Autodesk Inventor part; units mm, degrees
ref_plane "YZ Plane" through (0, 0, 0) normal (1, 0, 0) x (0, 1, 0)
ref_plane "XZ Plane" through (0, 0, 0) normal (0, 1, 0) x (-1, 0, 0)
ref_plane "XY Plane" through (0, 0, 0) normal (0, 0, 1) x (1, 0, 0)
sketch "Sketch1" plane through (0, 0, 0) normal (0, 1, 0) x (-1, 0, 0)
  line L0 (41.8301, 96.0131) -> (-38.1699, 96.0131)
  line L1 (-38.1699, 96.0131) -> (-38.1699, -53.9869)
  line L2 (-38.1699, -53.9869) -> (41.8301, -53.9869)
  line L3 (41.8301, -53.9869) -> (41.8301, 96.0131)
  line L4 (41.8301, 81.0131) -> (-35.1699, 81.0131)
  line L5 (-35.1699, 81.0131) -> (-35.1699, -38.9869)
  line L6 (-35.1699, -38.9869) -> (41.8301, -38.9869)
  line L7 (41.8301, -38.9869) -> (41.8301, 81.0131)
  point P0 (0, 0)
  dimension "d0" = 80
  dimension "d1" = 150
  dimension "d2" = 15
  dimension "d3" = 15
  dimension "d4" = 3
extrude "Extrusion1" add sketch "Sketch1" along normal blind 15 contours L3 L4 L5 L6 L2 L1 L0
sketch "Sketch2" plane through (0, 15, 0) normal (0, 1, 0) x (1, 0, 0)
  line L0 (-41.8301, -96.0131) -> (38.1699, -96.0131)
  line L1 (-38.8301, -96.0131) -> (35.1699, -96.0131)
  line L2 (35.1699, -96.0131) -> (35.1699, -85.0131)
  line L3 (35.1699, -85.0131) -> (-38.8301, -85.0131)
  line L4 (-38.8301, -85.0131) -> (-38.8301, -96.0131)
  line L5 (38.1699, 53.9869) -> (-41.8301, 53.9869)
  line L6 (-38.8301, 53.9869) -> (35.1699, 53.9869)
  line L7 (35.1699, 53.9869) -> (35.1699, 42.9869)
  line L8 (35.1699, 42.9869) -> (-38.8301, 42.9869)
  line L9 (-38.8301, 42.9869) -> (-38.8301, 53.9869)
  line L10 (35.1699, -81.0131) -> (-41.8301, -81.0131)
  line L11 (-41.8301, 38.9869) -> (35.1699, 38.9869)
  line L12 (-41.8301, 53.9869) -> (-41.8301, 38.9869)
  point P0 (0, 0)
  point P1 (35.1699, -96.0131)
  dimension "d7" = 4
  dimension "d8" = 4
  dimension "d9" = 3
extrude "Extrusion2" cut sketch "Sketch2" against normal blind 11
sketch "Sketch3" plane through (-41.8301, 0, -53.9869) normal (-1, 0, 0) x (0, 0, 1)
  circle A0 centre (5, 10) radius 1.4
  circle A1 centre (145, 10) radius 1.4
  line L0 (11, 15) -> (11, 4)
  line L1 (11, 4) -> (0, 4)
  line L2 (139, 15) -> (139, 4)
  line L3 (150, 4) -> (139, 4)
  point P0 (53.9869, 0)
  dimension "d12" = 2.8
  dimension "d13" = 2.8
  dimension "d14" = 6
  dimension "d15" = 6
  dimension "d16" = 6
  dimension "d17" = 6
extrude "Extrusion3" cut sketch "Sketch3" against normal through all
fillet "Fillet1" radius 1 5 edges at (-1.8301, 4, -42.9869) (-38.8301, 9.5, -42.9869) (-38.8301, 4, -48.4869) (35.1699, 4, -48.4869) (35.1699, 9.5, -42.9869)
fillet "Fillet2" radius 1 5 edges at (-38.8301, 9.5, 85.0131) (-38.8301, 4, 90.5131) (-1.8301, 4, 85.0131) (35.1699, 9.5, 85.0131) (35.1699, 4, 90.5131)
properties part number "leg_8u"
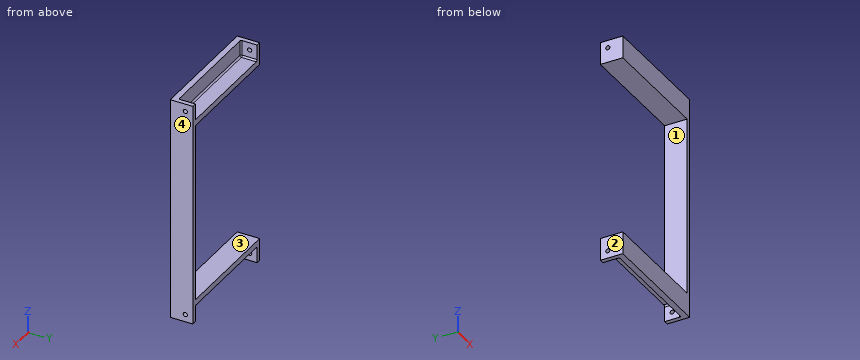
Build history of the part. All positions in model axes, mm. Face numbers are marked on the shaded views. A direction names the side the tool comes from. Round coordinates to 2 decimals unless told otherwise and drop trailing zeros. Loops run counter-clockwise (first coordinate to the right, second up) from the corner with the lowest first, then second, coordinate; pieces in that order, holes last. Notation, with made-up numbers: (49.5, 75.25) -> (101.5, 75.25) arc R34 ccw to (101.5, 106.25) -> close; hole circle Ø6 at (-36, 9.25). An arc over 180 degrees is marked (long way). One line per item, written item: value. Start each with the question number.
Q1. Drop flat-ended pins along their axis: pin 1 Ø1.5 at (y, z) = (13.5, -8) entering from -X; pin 2 Ø1 at (x, y) = (8.5, 8.5) entering from +Z; pin 3 Ø5 at (x, z) = (9, 89) entering from +Y; pin 4 Ø4.5 at (x, y) = (9, 5) entering from +Z. Give the stop position or say it passes through.
Q2. Cut at A-A on x = -5. List the corners of the cut face in (y, z), plus the area to 3 significant figures.
Q3. Cut at C-C on z = 38.5. List the corners of the cut face in (x, y), plus the area to 3 significant figures.
Q4. Probe line 1 along Z through (x, y) = (-20, 4.75); line 2 along X through (y, z) = (1, 22); line 3 along X through (y, z) = (6.75, -46). List the from-to ranges inside material, lowest first.
Q5. Two-plate mould, pull along Z, no slides. Class the marked faces 3 and 4: released by +Z, released by -Z, zero draft, split by the parting line, or undercut.
Q6. Cut at B-B on y = 6.5. List the corners of the cut face in (x, z).
Q7. 3-axis set-ups, long thin cutter, end or side, ignore diameter. For the marked faces 1 and 2: which of +Z, -Z, +X, -X, +Y, -Y reach the whole face in a straight line?
Computed:
1. pin 1: x = 35.17
1. pin 2: z = 85.01
1. pin 3: y = 4
1. pin 4: z = 96.01
2. outline: (0, -53.99) -> (4, -53.99) -> (4, -43.99) arc R1 cw to (5, -42.99) -> (15, -42.99) -> (15, -38.99) -> (0, -38.99) -> close; (0, 81.01) -> (15, 81.01) -> (15, 85.01) -> (5, 85.01) arc R1 cw to (4, 86.01) -> (4, 96.01) -> (0, 96.01) -> close
2. area: 208 mm²
3. outline: (35.17, 0) -> (38.17, 0) -> (38.17, 15) -> (35.17, 15) -> close
3. area: 45.0 mm²
4. line 1: -43.02 to -38.99, 81.01 to 85.04
4. line 2: 35.17 to 38.17
4. line 3: -41.83 to -38.83, 35.17 to 38.17
5. face 3: undercut
5. face 4: zero draft
6. outline: (-41.83, -53.99) -> (-38.83, -53.99) -> (-38.83, -43.99) arc R1 cw to (-37.83, -42.99) -> (34.17, -42.99) arc R1 cw to (35.17, -43.99) -> (35.17, -53.99) -> (38.17, -53.99) -> (38.17, 96.01) -> (35.17, 96.01) -> (35.17, 86.01) arc R1 cw to (34.17, 85.01) -> (-37.83, 85.01) arc R1 cw to (-38.83, 86.01) -> (-38.83, 96.01) -> (-41.83, 96.01) -> (-41.83, 81.01) -> (35.17, 81.01) -> (35.17, -38.99) -> (-41.83, -38.99) -> close
7. face 1: -X, +Y, -Y
7. face 2: +Z, -Z, -X, +Y, -Y
